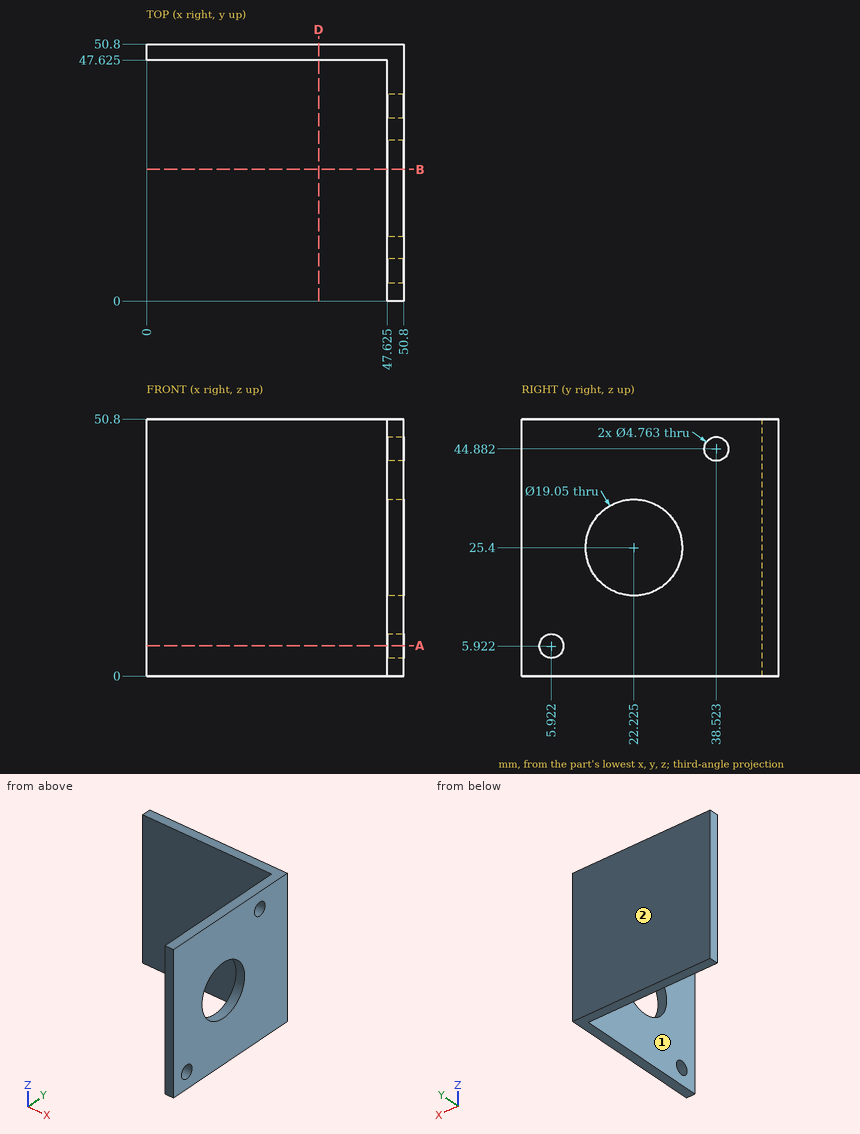
Can you work these out from the drawing? Everything is in mm from the part's minimum corner. A direction names the side the tool comes from. Round coordinates to 2 decimals unless told otherwise and drop trailing zeros. Write each loop counter-clockwise with the first axis right and the second up, starting at its lowest first coordinate (ties: lowest second). Pieces come first, ordered by that corner, then holes. Notation, with made-up numbers: (-18.5, 2.5) - (-0.5, 2.5) arc R22 ccw to (-0.5, 37.5) - close; hole circle Ø9 at (-27, 5.5). An arc over 180 degrees is marked (long way). Put each result on its own line as item: value. Start each with the question number.
(1) I want a section at A-A, the plane z = 6. Please give me the cut outline in (x, y) (1 decimal).
(2) I want a section at D-D, the plane x = 34. Please give me the cut outline in (y, z) (1 decimal), plus the area to 3 significant figures.
(3) I need wall thicknesses on probe 1 along Y at (x, z) = (49.15, 25.4); probe 2 along Y at (x, z) = (26, 22) (1 decimal). Which ranges of each line are inside material? Lowest first, please.
(4) For the marked faces 1 and 2, which set-ups out of +Z, -Z, +X, -X, +Y, -Y let a thin tool reach every point of the face, with its end or its side?
(5) I want a section at B-B, the plane y = 26. Please give me the cut outline in (x, z) (1 decimal).
(6) Will these pins go through, and if not, where does the flat tip stop? pin 1 (6 mm diameter, centred on y = 28.5, z = 13, fed in from -X) (3 decimals); pin 2 (5 mm diameter, centred on x = 7.5, z = 38.5, fed in from -Y) (3 decimals).
Here are the results:
1. outline: (0, 47.6) - (47.6, 47.6) - (47.6, 8.3) - (50.8, 8.3) - (50.8, 50.8) - (0, 50.8) - close; (47.6, 0) - (50.8, 0) - (50.8, 3.5) - (47.6, 3.5) - close
2. outline: (47.6, 0) - (50.8, 0) - (50.8, 50.8) - (47.6, 50.8) - close
2. area: 161 mm^2
3. probe 1: y = 0 to 12.7, 31.75 to 50.8
3. probe 2: y = 47.6 to 50.8
4. face 1: +Z, -Z, -X, -Y
4. face 2: +Z, -Z, +X, -X, +Y
5. outline: (47.6, 0) - (50.8, 0) - (50.8, 16.7) - (47.6, 16.7) - close; (47.6, 34.1) - (50.8, 34.1) - (50.8, 50.8) - (47.6, 50.8) - close
6. pin 1: stops at x = 47.625
6. pin 2: stops at y = 47.625
